The listing builds one solid part. Answer for the finished solid, in the listing's coordinates (mm). Give positions to 0.01 mm unless a question says otherwise; leave off trailing zeros. Order: outer loops, then holes, each group sorted by start corner. A loop starts at its lowest first (then second) coordinate and runs counter-clockwise, first axis right, second up.
```python
from build123d import *

# Parameters (mm, degrees)
BOSS_EXTRUDE1_DEPTH = 2
SKETCH4_W           = 1
SKETCH4_H           = 10
CUT_EXTRUDE1_DEPTH  = 124.438243669


with BuildPart() as part:
    # Sketch3 → Boss-Extrude1 (new body)
    with BuildSketch(Plane(origin=(0, 0, 0), x_dir=(1, 0, 0), z_dir=(0, 1, 0))):
        Polygon((-103, 0), (-103, 45), (-23, 68), (-18, 68), (-18, 26), (18, 26), (18, 68), (23, 68), (103, 45), (103, 0), align=None)
    extrude(amount=BOSS_EXTRUDE1_DEPTH)

    # Sketch4 → Cut-Extrude1 (cut, through all)
    with BuildSketch(Plane(origin=(0, 2, 0), x_dir=(1, 0, 0), z_dir=(0, 1, 0))):
        with Locations((-97.5, 7)):
            Rectangle(SKETCH4_W, SKETCH4_H)
        with Locations((-84.5, 7)):
            Rectangle(SKETCH4_W, SKETCH4_H)
        with Locations((-31.5, 7)):
            Rectangle(SKETCH4_W, SKETCH4_H)
        with Locations((-18.5, 7)):
            Rectangle(SKETCH4_W, SKETCH4_H)
    cut_extrude1 = extrude(amount=-CUT_EXTRUDE1_DEPTH, mode=Mode.SUBTRACT)

    # Mirror1: Cut-Extrude1 across plane
    add(cut_extrude1.mirror(Plane.ZY), mode=Mode.SUBTRACT)


solid = part.part
```
1) Given P1, Ø1.1, axis at x = 18.5, y = 1, coming from the +Z side; P2, Ø0.6, axis at x = 6.5, y = 1.5, coming from the -Z side; P3, Ø0.8, axis at x = 84.5, y = 1, coming from the -Z side, each flat-ended and moving along its own axis, determine where each tip first touches the part or whether it passes through.
Geometry says:
P1: stops at z = 0
P2: stops at z = -26
P3: stops at z = -50.43
2) For a pull along Z with two mould halves and no side action, classify faces 1 (the flat face through (62.44, 0.99, -56.66)), 2 (the flat face through (1, 2, -19)) as +Z half, -Z half, draft (parallel to the pull), parting line (faces both ways), or undercut.
Geometry says:
face 1: -Z half
face 2: draft
3) Find section A-A (z = -56.5). Write down the section's boundary in (x, y), then the cut area to 3 significant figures.
Geometry says:
outline: (-63, 0) - (-18, 0) - (-18, 2) - (-63, 2) - close; (18, 0) - (63, 0) - (63, 2) - (18, 2) - close
area: 180 mm2
4) Straight lines are drawn through the part: probe 1 along X at (y, z) = (1.75, -36); probe 2 along Z at (x, y) = (5, 0.9); probe 3 along Z at (x, y) = (-59, 0.25). For each, find the intervals that lie inside material, in ascending order.
Geometry says:
probe 1: x = -103 to -18, 18 to 103
probe 2: z = -26 to 0
probe 3: z = -57.65 to 0
5) Find section B-B (z = -30.5). Write down the section's boundary in (x, y).
Geometry says:
outline: (-103, 0) - (-18, 0) - (-18, 2) - (-103, 2) - close; (18, 0) - (103, 0) - (103, 2) - (18, 2) - close
6) Find section C-C (y = 0.3). Count the separate pieces of the cut face and the enclosed holes in it, then the cut area to 3 significant figures.
Geometry says:
separate pieces: 1
enclosed holes: 8
area: 10,600 mm2
